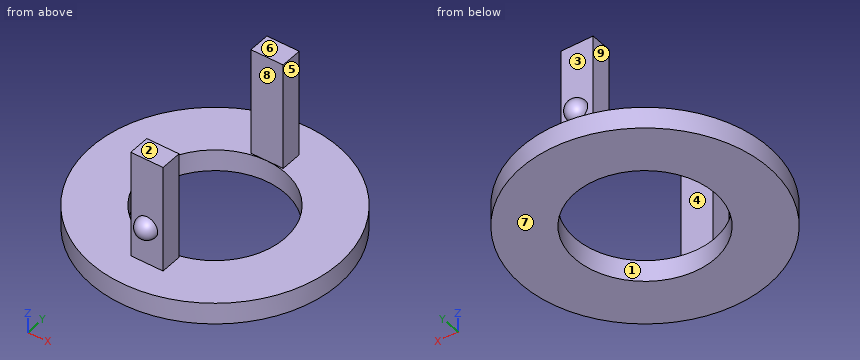
from build123d import *

# Parameters (mm, degrees)
SKETCH150_R         = 11.5
SKETCH150_R_2       = 6.5
PAD061_DEPTH        = 2
SKETCH151_W         = 3
SKETCH151_H         = 2
PAD062_DEPTH        = 10
REVOLUTION013_ANGLE = -180
REVOLUTION014_ANGLE = -180


with BuildPart() as part:
    # Sketch150 → Pad061 (new body)
    with BuildSketch(Plane.XY):
        Circle(SKETCH150_R)
        Circle(SKETCH150_R_2, mode=Mode.SUBTRACT)
    extrude(amount=PAD061_DEPTH)

    # Sketch151 (on Face4 of Pad061) → Pad062 (join)
    with BuildSketch(Plane.XY.offset(2)):
        with Locations((0, 7.5)):
            Rectangle(SKETCH151_W, SKETCH151_H)
        with Locations((0, -7.5)):
            Rectangle(SKETCH151_W, SKETCH151_H)
    extrude(amount=PAD062_DEPTH)

    # Sketch152 (on Face11 of Pad062) → Revolution013 (revolve)
    with BuildSketch(Plane.XZ.offset(8.5)):
        with BuildLine():
            ThreePointArc((0, 4.5), (1, 5.5), (0, 6.5))
            Line((0, 6.5), (0, 4.5))
        make_face()
    revolve(axis=Axis((0, -8.5, 0), (0, 0, 1)), revolution_arc=REVOLUTION013_ANGLE)

    # Sketch153 (on Face7 of Revolution013) → Revolution014 (revolve)
    with BuildSketch(Plane(origin=(0, 8.5, 0), x_dir=(-1, 0, 0), z_dir=(0, 1, 0))):
        with BuildLine():
            ThreePointArc((0, 4.5), (1, 5.5), (0, 6.5))
            Line((0, 6.5), (0, 4.5))
        make_face()
    revolve(axis=Axis((0, 8.5, 0), (0, 0, 1)), revolution_arc=REVOLUTION014_ANGLE)


solid = part.part
Here's how the part is built. I have some questions about the finished solid (model axes, mm). Face numbers are marked on the shaded views. A direction names the side the tool comes from. Give positions to 0.01 mm unless a question says otherwise; leave off trailing zeros. Loops run counter-clockwise (first coordinate to the right, second up) from the corner with the lowest first, then second, coordinate; pieces in that order, holes last. Notation, with made-up numbers: (21, 35.25) -> (35, 35.25) arc R21 cw to (35, 40.25) -> close; hole circle Ø7 at (60.25, 2). An arc over 180 degrees is marked (long way). Answer as a JSON object with one key per item and string values. Group by question number.
Item 1: I need wall thicknesses on L1, parallel to Y at x = -0.25, z = 2.75; L2, parallel to Y at x = 0, z = 0.65; L3, parallel to Z at x = 4.5, y = -9.5. Which ranges of each line are inside material? Lowest first, please.
Item 2: Imagine slicing it at A-A on z = 11.25. Write out the boundary of the cut face in (x, y), then the cut area to 3 significant figures.
Item 3: On a 3-axis mill with a long thin cutter (end or side, diameter ignored), from which of +Z, -Z, +X, -X, +Y, -Y can I reach the whole of each face in a straight line? I mean the marked faces 5, 6, 7, 8 and 9. Say none if no direction works.
Item 4: Imagine slicing it at D-D on y = 7. Write out the boundary of the cut face in (x, z).
Item 5: Will these pins go through, and if not, where does the flat tip stop? pin 1 (3.5 mm diameter, centred on x = 0.5, z = 4.5, fed in from -Y); pin 2 (1.5 mm diameter, centred on x = -0.5, z = 4.5, fed in from -Y); pin 3 (1 mm diameter, centred on y = -7.5, z = 4.5, fed in from +X).
Item 6: Imagine slicing it at C-C on z = 5.25. Write out the boundary of the cut face in (x, y).
Item 7: Thinking about a two-plate mould opening in Y: for the marked faces 1, 2, 3 and 4, which applies, pulls with the +Y half, pulls with the -Y half, needs draft (parallel to the pull), parting line crosses it, or undercut?
Item 8: Imagine slicing it at B-B on y = 0. Write out the boundary of the cut face in (x, z).
Answer list:
{
 "1": {"L1": "y = -8.5 to -6.5, 6.5 to 8.5", "L2": "y = -11.5 to -6.5, 6.5 to 11.5", "L3": "z = 0 to 2"},
 "2": {"outline": "(-1.5, -8.5) -> (1.5, -8.5) -> (1.5, -6.5) -> (-1.5, -6.5) -> close; (-1.5, 6.5) -> (1.5, 6.5) -> (1.5, 8.5) -> (-1.5, 8.5) -> close", "area": "12.0 mm2"},
 "3": {"face 5": "+Z, +X, +Y, -Y", "face 6": "+Z, +X, -X, +Y, -Y", "face 7": "-Z, +X, -X, +Y, -Y", "face 8": "+Z, +X, -X", "face 9": "+Z, -X, +Y, -Y"},
 "4": {"outline": "(-9.12, 0) -> (9.12, 0) -> (9.12, 2) -> (1.5, 2) -> (1.5, 12) -> (-1.5, 12) -> (-1.5, 2) -> (-9.12, 2) -> close"},
 "5": {"pin 1": "stops at y = -9.5", "pin 2": "stops at y = -9.43", "pin 3": "stops at x = 1.5"},
 "6": {"outline": "(-1.5, -8.5) -> (-0.97, -8.5) arc R0.97 ccw to (0.97, -8.5) -> (1.5, -8.5) -> (1.5, -6.5) -> (-1.5, -6.5) -> close; (-1.5, 6.5) -> (1.5, 6.5) -> (1.5, 8.5) -> (0.97, 8.5) arc R0.97 ccw to (-0.97, 8.5) -> (-1.5, 8.5) -> close"},
 "7": {"face 1": "undercut", "face 2": "needs draft", "face 3": "pulls with the +Y half", "face 4": "undercut"},
 "8": {"outline": "(-11.5, 0) -> (-6.5, 0) -> (-6.5, 2) -> (-11.5, 2) -> close; (6.5, 0) -> (11.5, 0) -> (11.5, 2) -> (6.5, 2) -> close"}
}
